from build123d import *

# Parameters (mm, degrees)
F1_DEPTH = 25.4
F2_DEPTH = 508


with BuildPart() as f1:
    # F0 (on Front) → F1 (new body)
    with BuildSketch(Plane.XZ):
        with BuildLine():
            Line((-23.26887446, 0), (23.26887446, 0))
            ThreePointArc((23.26887446, 0), (20.4736338233, 11.0576144219), (12.7594845956, 19.4585732131))
            Line((12.7594845956, 19.4585732131), (0.4321157806, 23.2648618003))
            Line((0.4321157806, 23.2648618003), (-13.2265486778, 19.1441617396))
            ThreePointArc((-13.2265486778, 19.1441617396), (-20.6059144344, 10.8091076855), (-23.26887446, 0))
        make_face()
        with BuildLine():
            Line((75.7796689868, 0), (23.26887446, 0))
            ThreePointArc((23.26887446, 0), (20.5584527971, -10.8991071756), (13.0586223544, -19.2590991701))
            Line((13.0586223544, -19.2590991701), (75.7796689868, 0))
        make_face()
        with BuildLine():
            ThreePointArc((12.7594845956, 19.4585732131), (20.4736338233, 11.0576144219), (23.26887446, 0))
            Line((23.26887446, 0), (75.7796689868, 0))
            Line((75.7796689868, 0), (12.7594845956, 19.4585732131))
        make_face()
        with BuildLine():
            ThreePointArc((13.0586223544, -19.2590991701), (20.5584527971, -10.8991071756), (23.26887446, 0))
            Line((23.26887446, 0), (-23.26887446, 0))
            ThreePointArc((-23.26887446, 0), (-20.5222893701, -10.9670487209), (-12.9309307101, -19.3450652521))
            Line((-12.9309307101, -19.3450652521), (0, -23.26887446))
            Line((0, -23.26887446), (13.0586223544, -19.2590991701))
        make_face()
        with BuildLine():
            Line((-76.6826793551, 0), (-23.26887446, 0))
            ThreePointArc((-23.26887446, 0), (-20.6059144344, 10.8091076855), (-13.2265486778, 19.1441617396))
            Line((-13.2265486778, 19.1441617396), (-76.6826793551, 0))
        make_face()
        with BuildLine():
            ThreePointArc((-12.9309307101, -19.3450652521), (-20.5222893701, -10.9670487209), (-23.26887446, 0))
            Line((-23.26887446, 0), (-76.6826793551, 0))
            Line((-76.6826793551, 0), (-12.9309307101, -19.3450652521))
        make_face()
    extrude(amount=F1_DEPTH)

    # F2 (add): a face of the model
    f2_faces = [f1.faces().sort_by_distance(p)[0] for p in [
        (-0.2289903697, -25.4, -0.0013375532),
    ]]
    extrude(f2_faces, amount=F2_DEPTH)


solid = f1.part
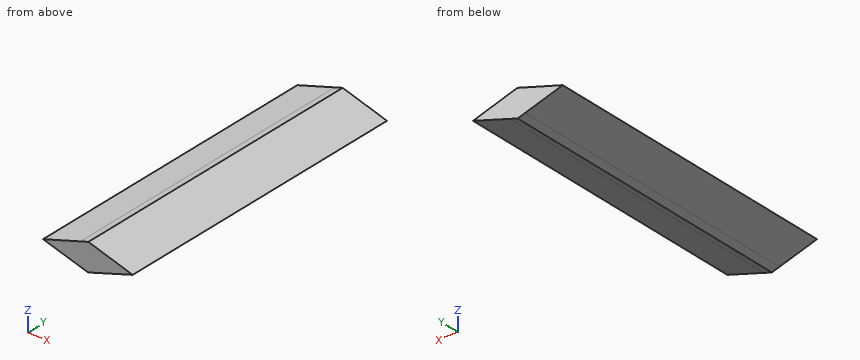
Input: part model. Units: mm. Frame: model coordinates. Coordinates: 2 decimals unless noted, no trailing zeros. Order: outer loops, then holes, each group sorted by start corner. A loop starts at its lowest first (then second) coordinate and runs counter-clockwise, first axis right, second up.
1. Ray query, line 1 along Z through (x, y) = (21, -41); line 2 along Z through (x, y) = (-20, -106.5). Return the intervals inside material, ascending.
Checked values:
line 1: z = -16.82 to 16.91
line 2: z = -17.2 to 17.1
2. Cut plane A-A, the plane y = -402.5. Return loops of the section in (x, z), plus the area to 3 significant figures.
Checked values:
outline: (-76.68, 0) - (0, -23.27) - (75.78, 0) - (0.43, 23.26) - close
area: 3,550 mm2
3. Contact query for flat-ended pins moving along their axis: P1, Ø6, axis at x = 50, y = -133.5, coming from the +Z side; P2, Ø3, axis at x = 53, y = -449.5, coming from the -Z side; P3, Ø1.5, axis at x = -3, y = -237, coming from the -Z side. Output: stop coordinate, or through.
Checked values:
P1: stops at z = 8.89
P2: stops at z = -7.46
P3: stops at z = -22.59
4. Cut plane C-C, the plane x = -49. Return loops of the section in (y, z), plus the area to 3 significant figures.
Checked values:
outline: (-533.4, -8.4) - (0, -8.4) - (0, 8.35) - (-533.4, 8.35) - close
area: 8,940 mm2
5. Cut plane B-B, the plane z = 6. Return loops of the section in (x, y), plus the area to 4 significant figures.
Checked values:
outline: (-56.79, -533.4) - (56.35, -533.4) - (56.35, 0) - (-56.79, 0) - close
area: 60,350 mm2
